Here's how the part is built. I have some questions about the finished solid (model axes, mm). A direction names the side the tool comes from. Round coordinates to 2 decimals unless told otherwise and drop trailing zeros. Write each loop counter-clockwise with the first axis right and the second up, starting at its lowest first coordinate (ties: lowest second). Pieces come first, ordered by that corner, then holes. Notation, with made-up numbers: (56, 40.25) -> (87, 40.25) arc R26 ccw to (87, 66.25) -> close; hole circle Ø11 at (38.5, -6). An arc over 180 degrees is marked (long way). Put each result on its own line as item: value. Start each with the question number.
1. Suppose I cut it at C-C (z = 15). Please give me the cut outline in (x, y), then the cut area to 3 significant figures.
2. We'd pull the mould along X, two halves only. Please class faces 1 (the face through (15, -3, -18)), 2 (the face through (0, -12, 10)), 3 (the face through (6, -18, 13)), 4 (the face through (60, -6, 3)): +X half, -X half, draft (parallel to the pull), parting line (faces both ways), or undercut.
3. Suppose I cut it at A-A (x = 55). Please give me the cut outline in (y, z), then the cut area to 3 significant figures.
4. Suppose I cut it at D-D (y = -5). Please give me the cut outline in (x, z), then the cut area to 3 significant figures.
5. Which directions (+Z, -Z, +X, -X, +Y, -Y) give clear straight access to the entire face, cutting with the end or side of a thin tool? Please do faces 5 (the face through (31, -12, 6)), 6 (the face through (25, -3, -6)), 7 (the face through (60, -19, 3)), 8 (the face through (18, -6, -7)).
6. For pin 1 (3 mm diameter, centred on y = -17.5, z = 20, fed in from -X); pin 2 (12 mm diameter, centred on y = -22, z = 21, fed in from +X); pin 3 (11.5 mm diameter, centred on y = -12.5, z = 18, fed in from -X); pin 4 (7.5 mm diameter, centred on x = 11, z = -9.5, fed in from -Y), each with a flat end and sliding along its axis, tell me the tip position at first contact or that it passes through.
7. Suppose I cut it at B-B (y = -11.5). Please give me the cut outline in (x, z), then the cut area to 3 significant figures.
8. I need wall thicknesses on probe 1 along Z at (x, y) = (12.5, -3.4); probe 2 along Z at (x, y) = (3.9, -12.5); probe 3 along Z at (x, y) = (32, -23.5). Which ranges of each line are inside material? Lowest first, please. Write a range as from..to.
```python
from build123d import *

# Parameters (mm, degrees)
F1_DEPTH  = 25
F3_DEPTH  = 6
F5_DEPTH  = 6
F6_R      = 6.5
F7_DEPTH  = 6
F8_W      = 25
F8_H      = 6
F9_DEPTH  = 24.5
F10_R     = 6.5
F11_DEPTH = 6


with BuildPart() as f1:
    # F0 (on Front) → F1 (new body)
    with BuildSketch(Plane.XZ):
        Polygon((0, 30.5), (0, 0), (70, 0), (70, 6), (6, 6), (6, 30.5), align=None)
    extrude(amount=F1_DEPTH)

    # F2 (on face) → F3 (cut)
    with BuildSketch(Plane.XY.offset(6)):
        with BuildLine():
            Line((70, -19), (70, -6))
            Line((70, -6), (50, -6))
            ThreePointArc((50, -6), (43.5, -12.5), (50, -19))
            Line((50, -19), (70, -19))
        make_face()
    extrude(amount=-F3_DEPTH, mode=Mode.SUBTRACT)

    # F4 (on face) → F5 (cut)
    with BuildSketch(Plane(origin=(0, 0, 0), x_dir=(0, -1, 0), z_dir=(-1, 0, 0))):
        with BuildLine():
            ThreePointArc((12.5, 30.5), (21.338835, 26.838835), (25, 18))
            Line((25, 18), (25, 30.5))
            Line((25, 30.5), (12.5, 30.5))
        make_face()
        with BuildLine():
            ThreePointArc((0, 18), (3.661165, 26.838835), (12.5, 30.5))
            Line((12.5, 30.5), (0, 30.5))
            Line((0, 30.5), (0, 18))
        make_face()
    extrude(amount=-F5_DEPTH, mode=Mode.SUBTRACT)

    # F6 (on face) → F7 (cut)
    with BuildSketch(Plane(origin=(0, 0, 0), x_dir=(0, -1, 0), z_dir=(-1, 0, 0))):
        with Locations((12.5, 18)):
            Circle(F6_R)
    extrude(amount=-F7_DEPTH, mode=Mode.SUBTRACT)

    # F8 (on face) → F9 (join)
    with BuildSketch(Plane(origin=(0, 0, 0), x_dir=(1, 0, 0), z_dir=(0, 0, -1))):
        with Locations((12.5, 3)):
            Rectangle(F8_W, F8_H)
    extrude(amount=F9_DEPTH)

    # F10 (on face) → F11 (cut)
    with BuildSketch(Plane.XZ.offset(6)):
        with BuildLine():
            ThreePointArc((12.5, -24.5), (3.661165, -20.838835), (0, -12))
            Line((0, -12), (0, -24.5))
            Line((0, -24.5), (12.5, -24.5))
        make_face()
        with BuildLine():
            ThreePointArc((25, -12), (21.338835, -20.838835), (12.5, -24.5))
            Line((12.5, -24.5), (25, -24.5))
            Line((25, -24.5), (25, -12))
        make_face()
        with Locations((12.5, -12)):
            Circle(F10_R)
    extrude(amount=-F11_DEPTH, mode=Mode.SUBTRACT)


solid = f1.part
```
Verdict:
1. outline: (0, -25) -> (6, -25) -> (6, -18.27) -> (0, -18.27) -> close; (0, -6.73) -> (6, -6.73) -> (6, 0) -> (0, 0) -> close
1. area: 80.8 mm^2
2. face 1: undercut
2. face 2: -X half
2. face 3: +X half
2. face 4: draft
3. outline: (-25, 0) -> (-19, 0) -> (-19, 6) -> (-25, 6) -> close; (-6, 0) -> (0, 0) -> (0, 6) -> (-6, 6) -> close
3. area: 72.0 mm^2
4. outline: (0, -12) arc R12.5 ccw to (12.5, -24.5) arc R12.5 ccw to (25, -12) -> (25, 0) -> (70, 0) -> (70, 6) -> (6, 6) -> (6, 28) -> (0, 28) -> close; hole circle Ø13 at (12.5, -12)
4. area: 965 mm^2
5. face 5: +Z, +X, +Y, -Y
5. face 6: -Z, +X, +Y, -Y
5. face 7: +Z, -Z, +X
5. face 8: -Z, +X, -X, -Y
6. pin 1: stops at x = 0
6. pin 2: stops at x = 6
6. pin 3: passes through
6. pin 4: stops at y = -6
7. outline: (0, 0) -> (43.58, 0) -> (43.58, 6) -> (6, 6) -> (6, 11.58) -> (0, 11.58) -> close; (0, 24.42) -> (6, 24.42) -> (6, 30.46) -> (0, 30.46) -> close
7. area: 331 mm^2
8. probe 1: z = -24.5..-18.5, -5.5..6
8. probe 2: z = 0..11.5, 24.5..30.5
8. probe 3: z = 0..6
